```python
from build123d import *

# Parameters (mm, degrees)
BOSS_EXTRUDE1_DEPTH = 10
CIRPATTERN1_COUNT   = 12
SKETCH2_R           = 2.5
BOSS_EXTRUDE2_DEPTH = 30
SKETCH6_W           = 1.5
SKETCH6_H           = 1.5
CUT_EXTRUDE1_DEPTH  = 4
CHAMFER2_SIZE       = 0.5
FILLET1_R           = 0.5
CHAMFER3_SIZE       = 0.1
FILLET2_R           = 0.5
SKETCH9_R           = 3.25
CUT_EXTRUDE2_DEPTH  = 1


with BuildPart() as part:
    # Sketch1 → Boss-Extrude1 (new body)
    with BuildSketch(Plane(origin=(0, 0, 0), x_dir=(0, 0, -1), z_dir=(1, 0, 0))):
        with BuildLine():
            Line((-0.645900046, 4.835422864), (-0.191806417, 6.920636512))
            ThreePointArc((-0.191806417, 6.920636512), (-0.157364247, 6.976799854), (-0.095460151, 6.999349067))
            ThreePointArc((-0.095460151, 6.999349067), (0, 7), (0.095460151, 6.999349067))
            ThreePointArc((0.095460151, 6.999349067), (0.157364247, 6.976799854), (0.191806417, 6.920636512))
            Line((0.191806417, 6.920636512), (0.645900046, 4.835422864))
            ThreePointArc((0.645900046, 4.835422864), (0.703017017, 4.733506728), (0.807327282, 4.680889089))
            ThreePointArc((0.807327282, 4.680889089), (0, -4.75), (-0.807327282, 4.680889089))
            ThreePointArc((-0.807327282, 4.680889089), (-0.703017017, 4.733506728), (-0.645900046, 4.835422864))
        make_face()
    boss_extrude1 = extrude(amount=BOSS_EXTRUDE1_DEPTH)

    # CirPattern1: Boss-Extrude1 ×12 about axis
    cirpattern1_axis = Axis((0, 0, 0), (1, 0, 0))
    for i in range(1, CIRPATTERN1_COUNT):
        add(boss_extrude1.rotate(cirpattern1_axis, i * 360 / CIRPATTERN1_COUNT))

    # Sketch2 → Boss-Extrude2 (add)
    with BuildSketch(Plane(origin=(10, 0, 0), x_dir=(0, 0, -1), z_dir=(1, 0, 0))):
        Circle(SKETCH2_R)
    extrude(amount=BOSS_EXTRUDE2_DEPTH)

    # Sketch6 → Revolve1 (revolve)
    with BuildSketch(Plane(origin=(0, 0, 0), x_dir=(1, 0, 0), z_dir=(0, 1, 0))):
        with Locations((29.25, 3.25)):
            Rectangle(SKETCH6_W, SKETCH6_H)
    revolve(axis=Axis((0, 0, 0), (1, 0, 0)))

    # Sketch8 → Cut-Extrude1 (cut)
    with BuildSketch(Plane(origin=(0, 2.5, 0), x_dir=(1, 0, 0), z_dir=(0, 1, 0))):
        with BuildLine():
            Line((37, -0.844273094), (33, -0.844273094))
            ThreePointArc((33, -0.844273094), (32, 0.155726906), (33, 1.155726906))
            Line((33, 1.155726906), (37, 1.155726906))
            ThreePointArc((37, 1.155726906), (38, 0.155726906), (37, -0.844273094))
        make_face()
    extrude(amount=-CUT_EXTRUDE1_DEPTH, mode=Mode.SUBTRACT)

    # Chamfer2
    chamfer2_edges = [part.edges().sort_by_distance(p)[0] for p in [
        (40, 0, 2.5),
    ]]
    chamfer(chamfer2_edges, length=CHAMFER2_SIZE)

    # Fillet1
    fillet1_edges = [part.edges().sort_by_distance(p)[0] for p in [
        (28.5, 0, 2.5),
        (30, 0, 2.5),
    ]]
    fillet(fillet1_edges, radius=FILLET1_R)

    # Chamfer3
    chamfer3_edges = [part.edges().sort_by_distance(p)[0] for p in [
        (30, 0, 4),
        (28.5, 0, 4),
    ]]
    chamfer(chamfer3_edges, length=CHAMFER3_SIZE)

    # Fillet2
    fillet2_edges = [part.edges().sort_by_distance(p)[0] for p in [
        (10, 0, 2.5),
    ]]
    fillet(fillet2_edges, radius=FILLET2_R)

    # Sketch9 → Cut-Extrude2 (cut)
    with BuildSketch(Plane.ZY):
        Circle(SKETCH9_R)
    extrude(amount=-CUT_EXTRUDE2_DEPTH, mode=Mode.SUBTRACT)


solid = part.part
```
Here's how the part is built. I have some questions about the finished solid (model axes, mm). A direction names the side the tool comes from. Give positions to 0.01 mm unless a question says otherwise; leave off trailing zeros. Loops run counter-clockwise (first coordinate to the right, second up) from the corner with the lowest first, then second, coordinate; pieces in that order, holes last. Notation, with made-up numbers: M -32,-32.75 L 17,-32.75 A28 ccw 17,-13.75 Z; hole C -6,40.25 d6. An arc over 180 degrees is marked long. Use one line per item in the form item = value. Start each with the question number.
Q1. Will these pins go through, and if not, where does the flat tip stop? pin 1 Ø4 at (x, z) = (21.5, -3) entering from +Y; pin 2 Ø3 at (y, z) = (-0.5, 1) entering from -X; pin 3 Ø1.6 at (x, z) = (34, 0.5) entering from +Y; pin 4 Ø4 at (y, z) = (2, -1.5) entering from +X.
Q2. Thinking about a two-plate mould opening in X: for faces 5 (the flat face through (35, 0, -1.156)), 6 (the flat face through (40, 0, 0)), 7 (the flat face through (4.93, 0.422, -5.863)), which applies, +X half, -X half, draft (parallel to the pull), parting line (faces both ways), or undercut?
Q3. Which directions (+Z, -Z, +X, -X, +Y, -Y) give clear straight access to the entire face, cutting with the end or side of a thin tool? Please do faces 1 (the flat face through (35, -1.5, 0)), 2 (the flat face through (4.93, -3.3, 4.87)), 3 (the flat face through (4.93, 5.863, 0.422)), 4 (the cylindrical face through (34.94, -2.44, 0.54)).
Q4. I need wall thicknesses on line 1 along Y through (x, z) = (0.6, 0); line 2 along Y through (x, z) = (7, 5); line 3 along X through (y, z) = (-4, -1). Which ranges of each line are inside material? Lowest first, please.
Q5. If we section it at A-A (x = 22): Write out the boundary of the cut face in (y, z), then the cut area to 3 significant figures.
Taken from the geometry:
q1.pin_1 = 2.29
q1.pin_2 = 1
q1.pin_3 = 2.35
q1.pin_4 = 40
q2.face_5 = undercut
q2.face_6 = +X half
q2.face_7 = draft
q3.face_1 = +Y
q3.face_2 = +X, -X, -Y
q3.face_3 = +X, -X, +Y
q3.face_4 = +X
q4.line_1 = -7 to -3.25, 3.25 to 7
q4.line_2 = -3.34 to -2.3, -0.61 to 0.61, 2.3 to 3.34
q4.line_3 = 0 to 10
q5.outline = C 0,0 d5
q5.area = 19.6 mm^2
